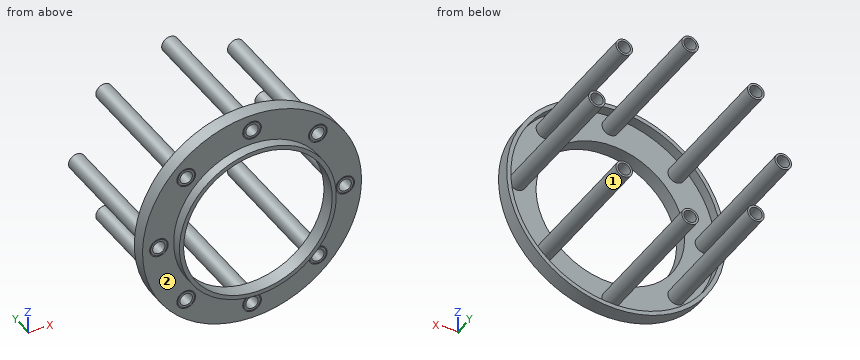
```python
from build123d import *

# Parameters (mm, degrees)
IZIM2_R                        = 4
KES_EKSTR_ZYON1_DEPTH          = 10
PAH1_SIZE                      = 0.5
DAIRESEL_KAPLAMA8_COUNT        = 8
PAH1_OF_DAIRESEL_KAPLAMA8_SIZE = 0.5
IZIM4_R                        = 4
IZIM4_R_2                      = 3
Y_KSEKLIK_EKSTR_ZYON2_DEPTH    = 70


with BuildPart() as part:
    # Çizim1 → Döndür1 (revolve)
    with BuildSketch(Plane.XY, mode=Mode.PRIVATE) as d_nd_r1_sk:
        Polygon((-52.9, 7), (-52.9, 0), (-37.9, 0), (-37.9, -5), (-35.9, -5), (-35.9, 2), (-50.9, 2), (-50.9, 7), align=None)
    revolve(d_nd_r1_sk.sketch.rotate(Axis((0, 0, 0), (0, 1, 0)), 270), axis=Axis((0, 0, 0), (0, 1, 0)))

    # Çizim2 → Kes-Ekstrüzyon1 (cut)
    with BuildSketch(Plane.XZ):
        with Locations(Location((0, 45, 0), (0, 0, 270))):
            Circle(IZIM2_R)
    kes_ekstr_zyon1 = extrude(amount=-KES_EKSTR_ZYON1_DEPTH, mode=Mode.SUBTRACT)

    # Pah1
    pah1_edges = [part.edges().sort_by_distance(p)[0] for p in [
        (0, 0, 49),
    ]]
    chamfer(pah1_edges, length=PAH1_SIZE)

    # Dairesel Kaplama8: Kes-Ekstrüzyon1 ×8 about axis
    dairesel_kaplama8_axis = Axis((0, 0, 0), (0, 1, 0))
    for i in range(1, DAIRESEL_KAPLAMA8_COUNT):
        add(kes_ekstr_zyon1.rotate(dairesel_kaplama8_axis, i * 360 / DAIRESEL_KAPLAMA8_COUNT), mode=Mode.SUBTRACT)

    # Pah1 of Dairesel Kaplama8
    pah1_of_dairesel_kaplama8_edges = [part.edges().sort_by_distance(p)[0] for p in [
        (34.648232278, 0, 34.648232278),
        (49, 0, 0),
        (34.648232278, 0, -34.648232278),
        (0, 0, -49),
        (-34.648232278, 0, -34.648232278),
        (-49, 0, 0),
        (-34.648232278, 0, 34.648232278),
    ]]
    chamfer(pah1_of_dairesel_kaplama8_edges, length=PAH1_OF_DAIRESEL_KAPLAMA8_SIZE)

    # Çizim4 → Yükseklik-Ekstrüzyon2 (add)
    # profile 1 of 8: a face of its own
    with BuildSketch(Plane.XZ):
        with Locations(Location((0, 45, 0), (0, 0, 270))):
            Circle(IZIM4_R)
        with Locations(Location((0, 45, 0), (0, 0, 270))):
            Circle(IZIM4_R_2, mode=Mode.SUBTRACT)
    # profile 2 of 8: a face of its own
    with BuildSketch(Plane.XZ):
        with Locations(Location((31.819805153, 31.819805153, 0), (0, 0, 270))):
            Circle(IZIM4_R)
        with Locations(Location((31.819805153, 31.819805153, 0), (0, 0, 270))):
            Circle(IZIM4_R_2, mode=Mode.SUBTRACT)
    # profile 3 of 8: a face of its own
    with BuildSketch(Plane.XZ):
        with Locations(Location((45, 0, 0), (0, 0, 270))):
            Circle(IZIM4_R)
        with Locations(Location((45, 0, 0), (0, 0, 270))):
            Circle(IZIM4_R_2, mode=Mode.SUBTRACT)
    # profile 4 of 8: a face of its own
    with BuildSketch(Plane.XZ):
        with Locations(Location((31.819805153, -31.819805153, 0), (0, 0, 270))):
            Circle(IZIM4_R)
        with Locations(Location((31.819805153, -31.819805153, 0), (0, 0, 270))):
            Circle(IZIM4_R_2, mode=Mode.SUBTRACT)
    # profile 5 of 8: a face of its own
    with BuildSketch(Plane.XZ):
        with Locations(Location((0, -45, 0), (0, 0, 270))):
            Circle(IZIM4_R)
        with Locations(Location((0, -45, 0), (0, 0, 270))):
            Circle(IZIM4_R_2, mode=Mode.SUBTRACT)
    # profile 6 of 8: a face of its own
    with BuildSketch(Plane.XZ):
        with Locations(Location((-31.819805153, -31.819805153, 0), (0, 0, 270))):
            Circle(IZIM4_R)
        with Locations(Location((-31.819805153, -31.819805153, 0), (0, 0, 270))):
            Circle(IZIM4_R_2, mode=Mode.SUBTRACT)
    # profile 7 of 8: a face of its own
    with BuildSketch(Plane.XZ):
        with Locations(Location((-45, 0, 0), (0, 0, 270))):
            Circle(IZIM4_R)
        with Locations(Location((-45, 0, 0), (0, 0, 270))):
            Circle(IZIM4_R_2, mode=Mode.SUBTRACT)
    # profile 8 of 8: a face of its own
    with BuildSketch(Plane.XZ):
        with Locations(Location((-31.819805153, 31.819805153, 0), (0, 0, 270))):
            Circle(IZIM4_R)
        with Locations(Location((-31.819805153, 31.819805153, 0), (0, 0, 270))):
            Circle(IZIM4_R_2, mode=Mode.SUBTRACT)
    extrude(amount=-Y_KSEKLIK_EKSTR_ZYON2_DEPTH)


solid = part.part
```
Design review of the part built by this model. Coordinates are the model's own, in mm. Face numbers are marked on the shaded views. Give positions to 0.01 mm unless a question says otherwise; leave off trailing zeros. Order: outer loops, then holes, each group sorted by start corner. A loop starts at its lowest first (then second) coordinate and runs counter-clockwise, first axis right, second up. Notation, with made-up numbers: (18, -25.75) - (73, -25.75) arc R27 ccw to (73, 11.25) - close; hole circle Ø7 at (46, 26.25). An arc over 180 degrees is marked (long way). Use a Markdown table: item, result. Add a question column.
(1) Add section A-A on y = 17. Give the number of separate pieces and of enclosed holes in the cut face, then the cut area to 3 significant figures.
(2) Clearance check with flat-ended pins moving along their axes: P1, Ø4, axis at x = 30, z = -30.5, coming from the -Y side; P2, Ø10, axis at x = 2, y = 24, coming from the -Z side; P3, Ø5.5, axis at x = -45, z = 0, coming from the +Y side; P4, Ø1.5, axis at x = -32, z = -21, coming from the +Y side. State where each tip first meets the part, or that it passes through.
(3) Add section B-B on x = -45. Give the boundary of the cut face in (y, z).
(4) Mouldability with a two-part tool opening along X and no side actions: class the marked faces 1 and 2 as +X half, -X half, draft (parallel to the pull), parting line (faces both ways), or undercut.
(5) Wall thickness on probe 1 along X at (y, z) = (3.65, 0); probe 2 along X at (y, z) = (36, 0); probe 3 along X at (y, z) = (22, -45): over which ranges is each line inside the solid? List them lowest first. Write a range as [from, to].
(6) Add section C-C on z = 10.5. Give the boundary of the cut face in (x, y), then the cut area to 3 significant figures.
(7) Add section D-D on x = 22. Give the boundary of the cut face in (y, z), then the cut area to 3 significant figures.
Report:
| question | item | result |
|---|---|---|
| 1 | separate pieces | 8 |
| 1 | enclosed holes | 8 |
| 1 | area | 176 mm² |
| 2 | P1 | stops at y = 0 |
| 2 | P2 | stops at z = -49 |
| 2 | P3 | passes through |
| 2 | P4 | stops at y = 2 |
| 3 | outline | (0, -27.81) - (7, -27.81) - (7, -23.79) - (2, -23.79) - (2, -4) - (70, -4) - (70, -3) - (0, -3) - (0, -4) - (0.5, -4) - (0, -4.5) - close; (0, 3) - (70, 3) - (70, 4) - (2, 4) - (2, 23.79) - (7, 23.79) - (7, 27.81) - (0, 27.81) - (0, 4.5) - (0.5, 4) - (0, 4) - close |
| 4 | face 1 | undercut |
| 4 | face 2 | draft |
| 5 | probe 1 | x = [-52.9, -50.9], [-49, -48], [-42, -41], [41, 42], [48, 49], [50.9, 52.9] |
| 5 | probe 2 | x = [-49, -48], [-42, -41], [41, 42], [48, 49] |
| 5 | probe 3 | x = [-4, -3], [3, 4] |
| 6 | outline | (-51.85, 0) - (-36.42, 0) - (-36.42, -5) - (-34.33, -5) - (-34.33, 2) - (-49.81, 2) - (-49.81, 7) - (-51.85, 7) - close; (34.33, -5) - (36.42, -5) - (36.42, 0) - (51.85, 0) - (51.85, 7) - (49.81, 7) - (49.81, 2) - (34.33, 2) - close |
| 6 | area | 111 mm² |
| 7 | outline | (-5, -30.86) - (0, -30.86) - (0, -48.11) - (7, -48.11) - (7, -45.9) - (2, -45.9) - (2, -28.37) - (-5, -28.37) - close; (-5, 28.37) - (2, 28.37) - (2, 45.9) - (7, 45.9) - (7, 48.11) - (0, 48.11) - (0, 30.86) - (-5, 30.86) - close |
| 7 | area | 126 mm² |
